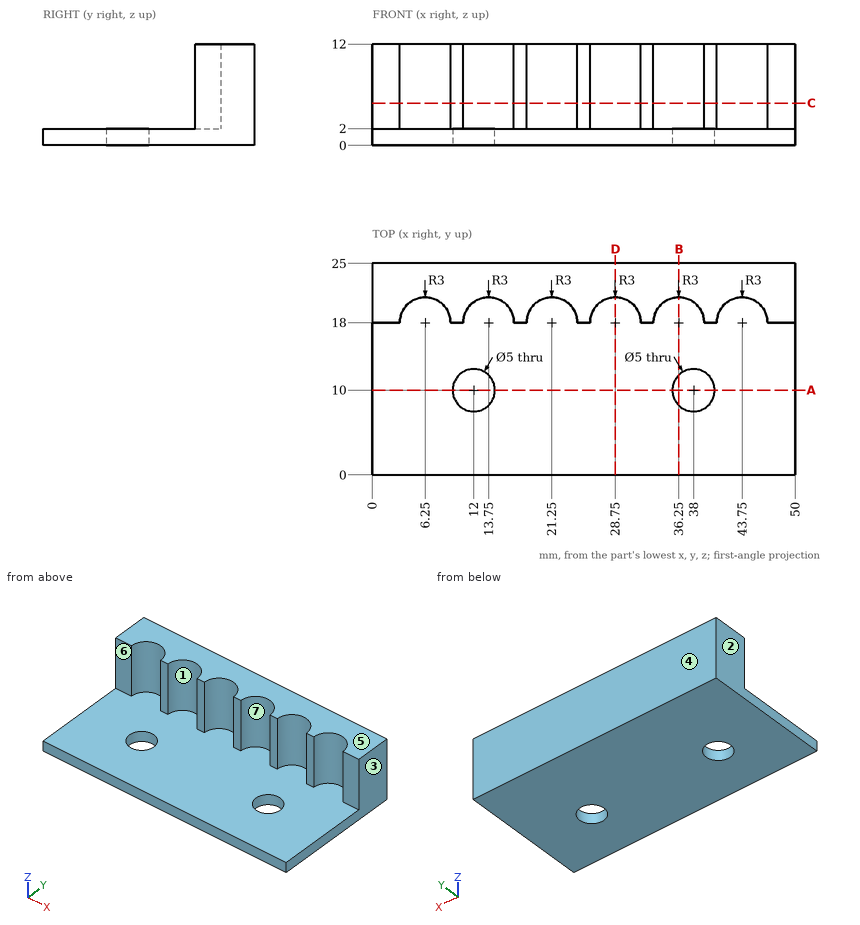
Part print with two shaded views. Sizes in mm from the minimum x, y, z corner. A direction names the side the tool comes from. Round coordinates to 2 decimals unless told otherwise and drop trailing zeros. Loops run counter-clockwise (first coordinate to the right, second up) from the corner with the lowest first, then second, coordinate; pieces in that order, holes last.
Item 1: Saw through at A-A (y = 10). List the corners of the cut face in (x, z), then the cut area to 3 significant figures.
Item 2: Which spindle directions (+Z, -Z, +X, -X, +Y, -Y) get a long thin tool onto all of the face, cutting with end or side? Do the marked faces 5, 6 and 7. Say none if no direction does.
Item 3: Two-plate mould, pull along X, no slides. Class the marked faces 1, 2, 3 and 4: released by +X, released by -X, zero draft, split by the parting line, or undercut.
Item 4: Saw through at D-D (x = 28.75). List the corners of the cut face in (y, z).
Item 5: Saw through at B-B (x = 36.25). List the corners of the cut face in (y, z).
Item 6: Drill centre lines: line 1 along Y through (x, z) = (38, 1); line 2 along Z through (x, y) = (44.5, 11.75); line 3 along Y through (x, z) = (32, 2.5). Where is each one in solid material? Low to high.
Item 7: Saw through at C-C (z = 5). List the corners of the cut face in (x, y), then the cut area to 3 significant figures.
Item 8: Pin check, flat tips, straight feed: P1, Ø1.2, axis at x = 25, z = 8, coming from the -Y side; P2, Ø6, axis at y = 20, z = 6, coming from the -X side; P3, Ø8, axis at x = 12, y = 10, coming from the +Z side. Stop position of each tip, or through.
Worked answers:
1. outline: (0, 0) - (9.5, 0) - (9.5, 2) - (0, 2) - close; (14.5, 0) - (35.5, 0) - (35.5, 2) - (14.5, 2) - close; (40.5, 0) - (50, 0) - (50, 2) - (40.5, 2) - close
1. area: 80.0 mm2
2. face 5: +Z, +X, -X, +Y, -Y
2. face 6: +Z, +X, -X, -Y
2. face 7: +Z, -Y
3. face 1: undercut
3. face 2: released by -X
3. face 3: released by +X
3. face 4: zero draft
4. outline: (0, 0) - (25, 0) - (25, 12) - (21, 12) - (21, 2) - (0, 2) - close
5. outline: (0, 0) - (8.21, 0) - (8.21, 2) - (0, 2) - close; (11.79, 0) - (25, 0) - (25, 12) - (21, 12) - (21, 2) - (11.79, 2) - close
6. line 1: y = 0 to 7.5, 12.5 to 25
6. line 2: z = 0 to 2
6. line 3: y = 18 to 25
7. outline: (0, 18) - (3.25, 18) arc R3 cw to (9.25, 18) - (10.75, 18) arc R3 cw to (16.75, 18) - (18.25, 18) arc R3 cw to (24.25, 18) - (25.75, 18) arc R3 cw to (31.75, 18) - (33.25, 18) arc R3 cw to (39.25, 18) - (40.75, 18) arc R3 cw to (46.75, 18) - (50, 18) - (50, 25) - (0, 25) - close
7. area: 265 mm2
8. P1: stops at y = 18
8. P2: stops at x = 0
8. P3: stops at z = 2
